Work out the finished part from the listing and answer in its coordinate system (mm). Coordinates: 2 decimals unless noted, no trailing zeros. Order: outer loops, then holes, each group sorted by start corner. A loop starts at its lowest first (then second) coordinate and runs counter-clockwise, first axis right, second up. Notation, with made-up numbers: M 26.25,24 L 50.25,24 A12 ccw 50.25,29 Z; hole C 52.5,12.25 d3. An arc over 180 degrees is marked long. Answer in a Markdown table with one row per item. Add a question column.
Item 1: Consider line 1 (Z direction, x = -17, y = -33.55); line 2 (Z direction, x = 0, y = -33.4); line 3 (Z direction, x = 15, y = -33). Determine where each line is inside the solid, lowest interval first. Write a range as from..to.
Item 2: A flat-ended cylindrical pin translates along its axis: pin 1 Ø3.5 at (x, z) = (-9.88, 1.95) entering from -Y. Find the tip coordinate at first contact, or state that the pin passes through.
Item 3: The part is cut by section A-A (z = 0.5). Write down the section's boundary in (x, y).
Item 4: The part is cut by section C-C (z = -11.5). Write down the section's boundary in (x, y).
Item 5: The part is cut by section D-D (z = 6). Write down the section's boundary in (x, y), then the cut area to 3 significant figures.
Item 6: The part is cut by section B-B (y = -33.6). State how many separate pieces and enclosed holes the cut face has, then the cut area to 3 significant figures.
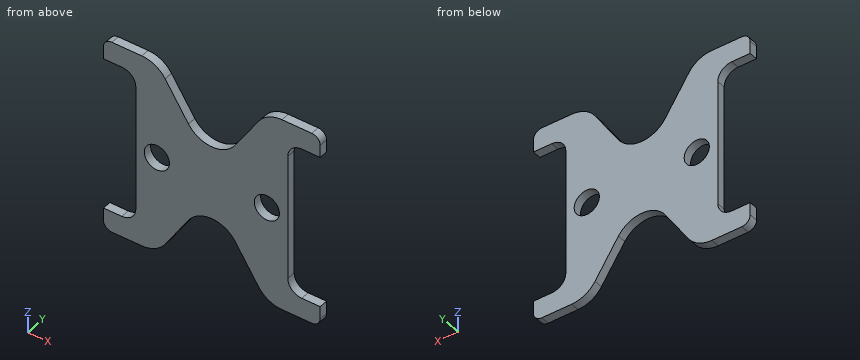
from build123d import *

# Parameters (mm, degrees)
SKETCH2_R           = 2.286
BOSS_EXTRUDE1_DEPTH = 1.5875
FILLET1_R           = 5.08
FILLET2_R           = 2.54
FILLET3_R           = 1.524


with BuildPart() as part:
    # Sketch2 → Boss-Extrude1 (new body)
    with BuildSketch(Plane.XZ.offset(32.657932219)):
        Polygon((10.109157694, -15.832760328), (13.919157694, -15.832760328), (19.794157694, -15.832760328), (19.794157694, -12.022760328), (13.919157694, -12.022760328), (13.919157694, 15.917239672), (19.794157694, 15.917239672), (19.794157694, 19.727239672), (13.919157694, 19.727239672), (10.109157694, 19.727239672), (0.109157694, 4.487239672), (-9.879450107, 19.727239672), (-13.700842306, 19.727239672), (-19.575842306, 19.727239672), (-19.575842306, 15.917239672), (-13.700842306, 15.917239672), (-13.700842306, -12.022760328), (-19.575842306, -12.022760328), (-19.575842306, -15.832760328), (-13.700842306, -15.832760328), (-9.879450107, -15.832760328), (0.109157694, -0.592760328), align=None)
        with Locations(Location((-9.879450107, 1.947239672, 0), (0, 0, 270))):
            Circle(SKETCH2_R, mode=Mode.SUBTRACT)
        with Locations(Location((10.109157694, 1.947239672, 0), (0, 0, 270))):
            Circle(SKETCH2_R, mode=Mode.SUBTRACT)
    extrude(amount=BOSS_EXTRUDE1_DEPTH)

    # Fillet1
    fillet1_edges = [part.edges().sort_by_distance(p)[0] for p in [
        (10.109157694, -33.451682219, 19.727239672),
        (10.109157694, -33.451682219, -15.832760328),
        (0.109157694, -33.451682219, -0.592760328),
        (-9.879450107, -33.451682219, -15.832760328),
        (-9.879450107, -33.451682219, 19.727239672),
        (0.109157694, -33.451682219, 4.487239672),
    ]]
    fillet(fillet1_edges, radius=FILLET1_R)

    # Fillet2
    fillet2_edges = [part.edges().sort_by_distance(p)[0] for p in [
        (13.919157694, -33.451682219, 15.917239672),
        (13.919157694, -33.451682219, -12.022760328),
        (-13.700842306, -33.451682219, -12.022760328),
        (-13.700842306, -33.451682219, 15.917239672),
    ]]
    fillet(fillet2_edges, radius=FILLET2_R)

    # Fillet3
    fillet3_edges = [part.edges().sort_by_distance(p)[0] for p in [
        (19.794157694, -33.451682219, 19.727239672),
        (19.794157694, -33.451682219, -15.832760328),
        (-19.575842306, -33.451682219, -15.832760328),
        (-19.575842306, -33.451682219, 19.727239672),
    ]]
    fillet(fillet3_edges, radius=FILLET3_R)


solid = part.part
Reply:
| question | item | result |
|---|---|---|
| 1 | line 1 | z = -15.83..-12.02, 15.92..19.73 |
| 1 | line 2 | z = -4.78..8.67 |
| 1 | line 3 | z = -15.83..-11.56, 15.46..19.73 |
| 2 | pin 1 | passes through |
| 3 | outline | M -13.7,-34.25 L -11.65,-34.25 L -11.65,-32.66 L -13.7,-32.66 Z; M -8.11,-34.25 L 8.34,-34.25 L 8.34,-32.66 L -8.11,-32.66 Z; M 11.88,-34.25 L 13.92,-34.25 L 13.92,-32.66 L 11.88,-32.66 Z |
| 4 | outline | M -14.7,-34.25 L -7.04,-34.25 L -7.04,-32.66 L -14.7,-32.66 Z; M 7.27,-34.25 L 14.92,-34.25 L 14.92,-32.66 L 7.27,-32.66 Z |
| 5 | outline | M -13.7,-34.25 L 13.92,-34.25 L 13.92,-32.66 L -13.7,-32.66 Z |
| 5 | area | 43.8 mm2 |
| 6 | separate pieces | 1 |
| 6 | enclosed holes | 2 |
| 6 | area | 761 mm2 |
